Here's how the part is built. I have some questions about the finished solid (model axes, mm). A direction names the side the tool comes from. Round coordinates to 2 decimals unless told otherwise and drop trailing zeros. Order: outer loops, then holes, each group sorted by start corner. A loop starts at its lowest first (then second) coordinate and runs counter-clockwise, first axis right, second up. Notation, with made-up numbers: (89, 23.5) - (142, 23.5) arc R25 ccw to (142, 52.5) - close; hole circle Ø2 at (50, 25). An arc over 180 degrees is marked (long way). Answer as a JSON object with one key per item and string values.
```python
from build123d import *

# Parameters (mm, degrees)
SKIZZE1_W                       = 9.5
SKIZZE1_H                       = 11.093
SKIZZE1_W_2                     = 8.7
SKIZZE1_H_2                     = 4.7
SKIZZE1_H_3                     = 5.193
AUFSATZ_LINEAR_AUSTRAGEN1_DEPTH = 19.7
AUFSATZ_LINEAR_AUSTRAGEN2_DEPTH = 2.3
SCHNITT_LINEAR_AUSTRAGEN1_DEPTH = 13.7
SKIZZE4_W                       = 13.3
SKIZZE4_H                       = 5.193
SCHNITT_LINEAR_AUSTRAGEN2_DEPTH = 0.4
AUFSATZ_LINEAR_AUSTRAGEN3_DEPTH = 14.1
AUFSATZ_LINEAR_START            = -9.5
AUFSATZ_LINEAR_AUSTRAGEN4_DEPTH = 9.5


with BuildPart() as part:
    # Skizze1 → Aufsatz-Linear austragen1 (new body)
    with BuildSketch(Plane(origin=(0, 0, 0), x_dir=(1, 0, 0), z_dir=(0, 1, 0))):
        with Locations((4.75, 5.5465)):
            Rectangle(SKIZZE1_W, SKIZZE1_H)
        with Locations((4.75, 2.75)):
            Rectangle(SKIZZE1_W_2, SKIZZE1_H_2, mode=Mode.SUBTRACT)
        with Locations((4.75, 8.0965)):
            Rectangle(SKIZZE1_W_2, SKIZZE1_H_3, mode=Mode.SUBTRACT)
    extrude(amount=AUFSATZ_LINEAR_AUSTRAGEN1_DEPTH)

    # Skizze2 → Aufsatz-Linear austragen2 (add)
    with BuildSketch(Plane.ZY):
        Polygon((-11.093, 0), (-8.093, 10.13), (-5.093, 0), align=None)
    aufsatz_linear_austragen2 = extrude(amount=AUFSATZ_LINEAR_AUSTRAGEN2_DEPTH)

    # Spiegeln1: Aufsatz-Linear austragen2 across plane
    add(aufsatz_linear_austragen2.mirror(Plane(origin=(4.75, 0, 0), x_dir=(0, 0, 1), z_dir=(1, 0, 0))))

    # Skizze3 → Schnitt-Linear austragen1 (cut)
    with BuildSketch(Plane.ZY.offset(2.3)):
        Polygon((-10.379677593, 1), (-5.806322407, 1), (-8.093, 8.721348004), align=None)
    extrude(amount=-SCHNITT_LINEAR_AUSTRAGEN1_DEPTH, mode=Mode.SUBTRACT)

    # Skizze4 → Schnitt-Linear austragen2 (cut)
    with BuildSketch(Plane.XZ):
        with Locations((4.75, -8.0965)):
            Rectangle(SKIZZE4_W, SKIZZE4_H)
    extrude(amount=-SCHNITT_LINEAR_AUSTRAGEN2_DEPTH, mode=Mode.SUBTRACT)

    # Skizze5 → Aufsatz-Linear austragen3 (add)
    with BuildSketch(Plane.ZY.offset(2.3)):
        Polygon((-20.977529946, -17.120508076), (-20.631119785, -17.320508076), (-10.631119785, 0), (-11.093, 0), align=None)
    extrude(amount=-AUFSATZ_LINEAR_AUSTRAGEN3_DEPTH)

    # Skizze6 → Aufsatz-Linear austragen4 (add)
    with BuildSketch(Plane.ZY.offset(AUFSATZ_LINEAR_START)):
        Polygon((-20.977529946, -17.120508076), (-11.093, 0), (-11.093, 14.7), align=None)
    extrude(amount=AUFSATZ_LINEAR_AUSTRAGEN4_DEPTH)


solid = part.part
```
1. If I drill on L1, parallel to X at y = 4.5, z = -5; L2, parallel to Z at x = 2.5, y = 3; L3, parallel to Z at x = 5.5, y = 1, over which ranges is the centre line in solid material (lowest first)? Write a range as [from, to].
Responses:
{"L1": "[0, 0.4], [9.1, 9.5]", "L2": "[-14.73, -10.69], [-5.5, -5.1], [-0.4, 0]", "L3": "[-15.35, -10.69], [-5.5, -5.1], [-0.4, 0]"}
2. Thinking about a two-plate mould opening in Y: for faces 1 (the face through (5, 10, -5.1)), 2 (the face through (-1.134, 4.994, -9.614)), 3 (the face through (10.234, 4.807, -6.934)), which applies, pulls with the +Y half, pulls with the -Y half, needs draft (parallel to the pull), parting line crosses it, or undercut?
Responses:
{"face 1": "needs draft", "face 2": "pulls with the +Y half", "face 3": "undercut"}
3. Imagine slicing it at D-D (y = 9.5). List the corners of the cut face in (x, z) for me.
Responses:
{"outline": "(-2.3, -8.28) - (0, -8.28) - (0, -12.71) - (9.5, -12.71) - (9.5, -8.28) - (11.8, -8.28) - (11.8, -7.91) - (9.5, -7.91) - (9.5, 0) - (0, 0) - (0, -7.91) - (-2.3, -7.91) - close; hole (0.4, -10.69) - (9.1, -10.69) - (9.1, -5.5) - (0.4, -5.5) - close; hole (0.4, -5.1) - (9.1, -5.1) - (9.1, -0.4) - (0.4, -0.4) - close"}
4. For faces 4 (the face through (10.634, 4.994, -9.614)), 5 (the face through (0.4, 10, -3)), 6 (the face through (10.23, 4.91, -9.22)), 7 (the face through (5, 17, -11.093)), which set-ups out of +Z, -Z, +X, -X, +Y, -Y let a thin tool reach every point of the face, with its end or its side?
Responses:
{"face 4": "-Z, +X, +Y", "face 5": "+Y, -Y", "face 6": "-X", "face 7": "-Z, +X, -X, +Y"}
5. Imagine slicing it at B-B (x = 11). List the corners of the cut face in (y, z) for me, plus the area to 3 significant figures.
Responses:
{"outline": "(-17.32, -20.63) - (-17.12, -20.98) - (0, -11.09) - (10.13, -8.09) - (0, -5.09) - (0, -5.5) - (0.4, -5.5) - (0.4, -10.69) - (0, -10.69) - (0, -10.63) - close; hole (1, -10.38) - (8.72, -8.09) - (1, -5.81) - close", "area": "18.6 mm2"}
6. Imagine slicing it at C-C (z = -8.5). List the corners of the cut face in (x, y) for me, plus the area to 3 significant figures.
Responses:
{"outline": "(-2.3, 0) - (-1.9, 0) - (-1.9, 0.4) - (0.4, 0.4) - (0.4, 1) - (-2.3, 1) - close; (-2.3, 7.35) - (0.4, 7.35) - (0.4, 19.7) - (0, 19.7) - (0, 8.76) - (-2.3, 8.76) - close; (9.1, 0.4) - (11.4, 0.4) - (11.4, 0) - (11.8, 0) - (11.8, 8.76) - (9.5, 8.76) - (9.5, 19.7) - (9.1, 19.7) - (9.1, 7.35) - (11.4, 7.35) - (11.4, 1) - (9.1, 1) - close", "area": "22.5 mm2"}
7. For P1, Ø2.5, axis at x = 3, y = 9.5, coming from the +Z side; P2, Ø8, axis at y = 7, z = -15, coming from the +X side; P3, Ø1.8, axis at x = 10.5, z = -8.5, coming from the +Y side; P4, Ø2.5, axis at y = 14.5, z = -9, coming from the -X side, each with a flat end and sliding along its axis, tell me the tip position at first contact or that it passes through.
Responses:
{"P1": "z = 0", "P2": "x = 9.5", "P3": "y = 10.13", "P4": "x = 0"}
8. Imagine slicing it at A-A (x = 5). List the corners of the cut face in (y, z) for me, plus the area to 3 significant figures.
Responses:
{"outline": "(-17.32, -20.63) - (-17.12, -20.98) - (14.7, -11.09) - (19.7, -11.09) - (19.7, -10.69) - (0, -10.69) - (0, -10.63) - close; (0, -5.5) - (19.7, -5.5) - (19.7, -5.1) - (0, -5.1) - close; (0, -0.4) - (19.7, -0.4) - (19.7, 0) - (0, 0) - close", "area": "104 mm2"}
